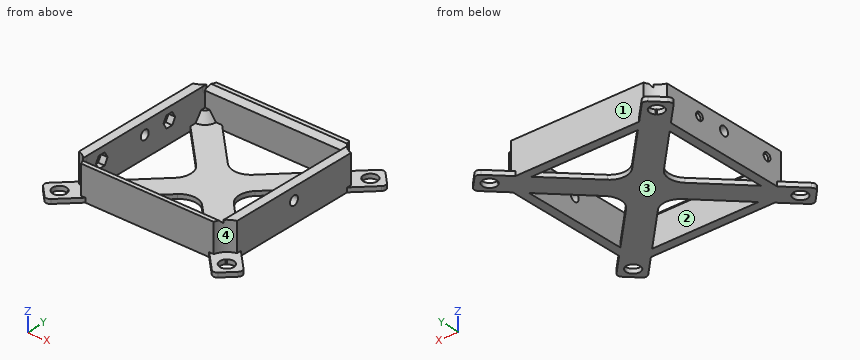
from build123d import *

# Parameters (mm, degrees)
CYLINDER_R               = 2.1
CYLINDER_DEPTH           = 73
PRISM_DEPTH              = 64
PRISM_ROLL_ANGLE         = 90
PRISM_PITCH_ANGLE        = -14.999988
PRISM_PLACEMENT_ANGLE    = 90
PRISM001_DEPTH           = 64
PRISM001_ROLL_ANGLE      = -90
PRISM001_PITCH_ANGLE     = -14.999988
PRISM001_PLACEMENT_ANGLE = -90
PRISM002_DEPTH           = 3
PRISM003_DEPTH           = 3
CYLINDER001_R            = 1.8
CYLINDER001_DEPTH        = 6
CYLINDER002_R            = 1.8
CYLINDER002_DEPTH        = 6
CUBE001_W                = 64
CUBE001_H                = 64
CUBE001_DEPTH            = 15
CUBE_W                   = 72
CUBE_H                   = 72
CUBE_DEPTH               = 15
SKETCH001_R              = 3.175
PAD_DEPTH                = 2
SKETCH_R                 = 8.125
POCKET_DEPTH             = 13
REVOLUTION_ANGLE         = -90


with BuildPart() as cylinder:
    # cylinder → cylinder (new body)
    with BuildSketch(Plane(origin=(-36.5, 0, -7.5), x_dir=(0, 1, 0), z_dir=(1, 0, 0))):
        Circle(CYLINDER_R)
    extrude(amount=CYLINDER_DEPTH)


with BuildPart() as prism:
    # prism → prism (new body)
    with BuildSketch(Plane.XY):
        Polygon((3, 0), (-1.5, 2.598076), (-1.5, -2.598076), align=None)
    extrude(amount=PRISM_DEPTH)


with BuildPart() as prism_1:
    # prism roll: moved
    add(prism.part.rotate(Axis((0, 0, 0), (1, 0, 0)), PRISM_ROLL_ANGLE))


with BuildPart() as prism_2:
    # prism pitch: moved
    add(prism_1.part.rotate(Axis((0, 0, 0), (0, 1, 0)), PRISM_PITCH_ANGLE))


with BuildPart() as prism_3:
    # prism placement: moved
    add(prism_2.part.moved(Location((-32.000004, 32, -2))).rotate(Axis((-32.000004, 32, -2), (0, 0, 1)), PRISM_PLACEMENT_ANGLE))


with BuildPart() as prism001:
    # prism001 → prism001 (new body)
    with BuildSketch(Plane.XY):
        Polygon((3, 0), (-1.5, 2.598076), (-1.5, -2.598076), align=None)
    extrude(amount=PRISM001_DEPTH)


with BuildPart() as prism001_1:
    # prism001 roll: moved
    add(prism001.part.rotate(Axis((0, 0, 0), (1, 0, 0)), PRISM001_ROLL_ANGLE))


with BuildPart() as prism001_2:
    # prism001 pitch: moved
    add(prism001_1.part.rotate(Axis((0, 0, 0), (0, 1, 0)), PRISM001_PITCH_ANGLE))


with BuildPart() as prism001_3:
    # prism001 placement: moved
    add(prism001_2.part.moved(Location((-32.000004, -32, -2))).rotate(Axis((-32.000004, -32, -2), (0, 0, 1)), PRISM001_PLACEMENT_ANGLE))


with BuildPart() as prism002:
    # prism002 → prism002 (new body)
    with BuildSketch(Plane(origin=(-35, 13.05, -7.5), x_dir=(0, 1, 0), z_dir=(1, 0, 0))):
        Polygon((3.1, 0), (1.55, 2.684679), (-1.55, 2.684679), (-3.1, 0), (-1.55, -2.684679), (1.55, -2.684679), align=None)
    extrude(amount=PRISM002_DEPTH)


with BuildPart() as prism003:
    # prism003 → prism003 (new body)
    with BuildSketch(Plane(origin=(-35, -22.85, -7.5), x_dir=(0, 1, 0), z_dir=(1, 0, 0))):
        Polygon((3.1, 0), (1.55, 2.684679), (-1.55, 2.684679), (-3.1, 0), (-1.55, -2.684679), (1.55, -2.684679), align=None)
    extrude(amount=PRISM003_DEPTH)


with BuildPart() as cylinder001:
    # cylinder001 → cylinder001 (new body)
    with BuildSketch(Plane(origin=(-36.5, 13.05, -7.5), x_dir=(0, 1, 0), z_dir=(1, 0, 0))):
        Circle(CYLINDER001_R)
    extrude(amount=CYLINDER001_DEPTH)


with BuildPart() as cylinder002:
    # cylinder002 → cylinder002 (new body)
    with BuildSketch(Plane(origin=(-36.5, -22.85, -7.5), x_dir=(0, 1, 0), z_dir=(1, 0, 0))):
        Circle(CYLINDER002_R)
    extrude(amount=CYLINDER002_DEPTH)


with BuildPart() as group:
    # cube001 → cube001 (new body)
    with BuildSketch(Plane(origin=(-32, -32, -17), x_dir=(1, 0, 0), z_dir=(0, 0, 1))):
        with Locations((32, 32)):
            Rectangle(CUBE001_W, CUBE001_H)
    extrude(amount=CUBE001_DEPTH)

    # Group: union cylinder, prism, prism001, prism002, prism003, cylinder001, cylinder002
    add(cylinder.part)
    add(prism_3.part)
    add(prism001_3.part)
    add(prism002.part)
    add(prism003.part)
    add(cylinder001.part)
    add(cylinder002.part)


with BuildPart() as base_square:
    # cube → cube (new body)
    with BuildSketch(Plane(origin=(-36, -36, -17), x_dir=(1, 0, 0), z_dir=(0, 0, 1))):
        with Locations((36, 36)):
            Rectangle(CUBE_W, CUBE_H)
    extrude(amount=CUBE_DEPTH)

    # difference: cut Group
    add(group.part, mode=Mode.SUBTRACT)

    # Sketch001 → Pad (new body)
    with BuildSketch(Plane(origin=(0, 0, -17), x_dir=(1, 0, 0), z_dir=(0, 0, -1))):
        with BuildLine():
            Line((-44.463961, 36.685786), (-13.435029, 5.656854))
            ThreePointArc((-13.435029, -5.656854), (-11.091883, 0), (-13.435029, 5.656854))
            Line((-13.435029, -5.656854), (-44.463961, -36.685786))
            ThreePointArc((-44.463961, -36.685786), (-45.049747, -38.1), (-44.463961, -39.514214))
            Line((-44.463961, -39.514214), (-39.514214, -44.463961))
            ThreePointArc((-39.514214, -44.463961), (-38.1, -45.049747), (-36.685786, -44.463961))
            Line((-36.685786, -44.463961), (-5.656854, -13.435029))
            ThreePointArc((5.656854, -13.435029), (0, -11.091883), (-5.656854, -13.435029))
            Line((5.656854, -13.435029), (36.685786, -44.463961))
            ThreePointArc((36.685786, -44.463961), (38.1, -45.049747), (39.514214, -44.463961))
            Line((39.514214, -44.463961), (44.463961, -39.514214))
            ThreePointArc((44.463961, -39.514214), (45.049747, -38.1), (44.463961, -36.685786))
            Line((44.463961, -36.685786), (13.435029, -5.656854))
            ThreePointArc((13.435029, 5.656854), (11.091883, 0), (13.435029, -5.656854))
            Line((13.435029, 5.656854), (44.463961, 36.685786))
            ThreePointArc((44.463961, 36.685786), (45.049747, 38.1), (44.463961, 39.514214))
            Line((44.463961, 39.514214), (39.514214, 44.463961))
            ThreePointArc((39.514214, 44.463961), (38.1, 45.049747), (36.685786, 44.463961))
            Line((36.685786, 44.463961), (5.656854, 13.435029))
            ThreePointArc((-5.656854, 13.435029), (0, 11.091883), (5.656854, 13.435029))
            Line((-5.656854, 13.435029), (-36.685786, 44.463961))
            ThreePointArc((-36.685786, 44.463961), (-38.1, 45.049747), (-39.514214, 44.463961))
            Line((-39.514214, 44.463961), (-44.463961, 39.514214))
            ThreePointArc((-44.463961, 39.514214), (-45.049747, 38.1), (-44.463961, 36.685786))
        make_face()
        with Locations((-38.1, 38.1)):
            Circle(SKETCH001_R, mode=Mode.SUBTRACT)
        with Locations((38.1, 38.1)):
            Circle(SKETCH001_R, mode=Mode.SUBTRACT)
        with Locations((-38.1, -38.1)):
            Circle(SKETCH001_R, mode=Mode.SUBTRACT)
        with Locations((38.1, -38.1)):
            Circle(SKETCH001_R, mode=Mode.SUBTRACT)
    extrude(amount=-PAD_DEPTH)

    # Sketch (on Face21 of Pad) → Pocket (cut)
    with BuildSketch(Plane.XY.offset(-2)):
        with Locations((-38.1, -38.1)):
            Circle(SKETCH_R)
        with Locations((38.1, -38.1)):
            Circle(SKETCH_R)
        with Locations((38.1, 38.1)):
            Circle(SKETCH_R)
        with Locations((-38.1, 38.1)):
            Circle(SKETCH_R)
    extrude(amount=-POCKET_DEPTH, mode=Mode.SUBTRACT)

    # Sketch002 (on Face26 of Pocket) → Revolution (revolve)
    with BuildSketch(Plane.XZ.offset(-32)):
        Polygon((-32, -15), (-32, -11), (-30, -11), (-27, -15), align=None)
    revolve(axis=Axis((-32, 32, -9.56066), (0, 0, 1)), revolution_arc=REVOLUTION_ANGLE)


solid = base_square.part
Verification items for the finished model (mm, model axes). Face numbers are marked on the shaded views. Give positions to 0.01 mm unless a question says otherwise; leave off trailing zeros. Loops run counter-clockwise (first coordinate to the right, second up) from the corner with the lowest first, then second, coordinate; pieces in that order, holes last.
1) Sectioned sample at A-A, the plane y = 0. Enter the section's corners in (x, z).
2) Sectioned sample at B-B, the plane x = 38.1. Enter the section's corners in (y, z) (3 decimals).
3) Thickness scan on line 1 along X through (y, z) = (2.5, -12); line 2 along Y through (x, z) = (38.1, -16.1) (3 decimals). Record the ranges inside material, lowest first.
4) Depth check by flat-ended pin: pin 1 Ø1.8 at (y, z) = (31, -3) entering from +X; pin 2 Ø4 at (x, z) = (-4, -11.5) entering from -Y; pin 3 Ø4 at (x, y) = (38.1, -38.1) entering from -Z (3 decimals); pin 4 Ø0.8 at (y, z) = (-32.5, -3.5) entering from -X. Enter the tip coordinate at first touch or a pass-through.
5) Sectioned sample at D-D, the plane y = 20. Enter the section's corners in (x, z).
6) Draft check along Y on the marked faces 1, 2, 3 and 4. Enter one of: pulls with the +Y half, pulls with the -Y half, needs draft (parallel to the pull), parting line crosses it, or undercut.
Answers:
1. outline: (-36, -17) - (-32, -17) - (-32, -9.6) - (-36, -9.6) - close; (-36, -5.4) - (-32, -5.4) - (-32, -2) - (-36, -2) - close; (-11.09, -17) - (11.09, -17) - (11.09, -15) - (-11.09, -15) - close; (32, -17) - (36, -17) - (36, -9.6) - (32, -9.6) - close; (32, -5.4) - (36, -5.4) - (36, -2) - (32, -2) - close
2. outline: (-45.05, -17) - (-41.275, -17) - (-41.275, -15) - (-45.05, -15) - close; (-34.925, -17) - (-30.322, -17) - (-30.322, -15) - (-34.925, -15) - close; (30.322, -17) - (34.925, -17) - (34.925, -15) - (30.322, -15) - close; (41.275, -17) - (45.05, -17) - (45.05, -15) - (41.275, -15) - close
3. line 1: x = -36 to -32, 32 to 36
3. line 2: y = -45.05 to -41.275, -34.925 to -30.322, 30.322 to 34.925, 41.275 to 45.05
4. pin 1: stops at x = 36
4. pin 2: stops at y = -36
4. pin 3: passes through
4. pin 4: stops at x = -32.62
5. outline: (-36, -17) - (-32, -17) - (-32, -2) - (-36, -2) - close; (-27.78, -17) - (-12.22, -17) - (-12.22, -15) - (-27.78, -15) - close; (12.22, -17) - (27.78, -17) - (27.78, -15) - (12.22, -15) - close; (32, -17) - (36, -17) - (36, -2) - (32, -2) - close
6. face 1: pulls with the +Y half
6. face 2: undercut
6. face 3: needs draft
6. face 4: pulls with the -Y half
